Verification items for the finished model (mm, model axes). A direction names the side the tool comes from. Give positions to 0.01 mm unless a question says otherwise; leave off trailing zeros. Write each loop counter-clockwise with the first axis right and the second up, starting at its lowest first coordinate (ties: lowest second). Pieces come first, ordered by that corner, then holes. Notation, with made-up numbers: (17, 7.5) -> (36, 7.5) arc R18 cw to (36, 28.5) -> close; hole circle Ø8 at (0.5, 55.5). An arc over 180 degrees is marked (long way). Answer as CSV lines item,"result".
```python
from build123d import *

# Parameters (mm, degrees)
SKETCH1_R           = 2
BOSS_EXTRUDE1_DEPTH = 6


with BuildPart() as part:
    # Sketch1 → Boss-Extrude1 (new body)
    with BuildSketch(Plane(origin=(0, 0, 0), x_dir=(1, 0, 0), z_dir=(0, 1, 0))):
        Polygon((-45, 15), (-45, -10), (-50, -10), (-50, -15), (-45, -15), (-45, -20), (-50, -20), (-50, -30), (-45, -30), (-45, -35), (-50, -35), (-50, -40), (-45, -40), (45, -40), (50, -40), (50, -35), (45, -35), (45, -33), (45, -30), (50, -30), (50, -20), (45, -20), (45, -15), (50, -15), (50, -10), (45, -10), (45, 15), (19, 35), (-19, 35), align=None)
        with Locations(Location((15, 0, 0), (0, 0, 270))):
            Circle(SKETCH1_R, mode=Mode.SUBTRACT)
        with Locations(Location((-15, 0, 0), (0, 0, 270))):
            Circle(SKETCH1_R, mode=Mode.SUBTRACT)
        with Locations(Location((15, 27, 0), (0, 0, 270))):
            Circle(SKETCH1_R, mode=Mode.SUBTRACT)
        with Locations(Location((-15, 27, 0), (0, 0, 270))):
            Circle(SKETCH1_R, mode=Mode.SUBTRACT)
        with Locations(Location((0, 30, 0), (0, 0, 270))):
            Circle(SKETCH1_R, mode=Mode.SUBTRACT)
        with Locations(Location((-36, -12, 0), (0, 0, 270))):
            Circle(SKETCH1_R, mode=Mode.SUBTRACT)
        with Locations(Location((36, -12, 0), (0, 0, 270))):
            Circle(SKETCH1_R, mode=Mode.SUBTRACT)
        with BuildLine():
            Line((7, -30.5), (23, -30.5))
            ThreePointArc((23, -30.5), (25.5, -33), (23, -35.5))
            Line((23, -35.5), (7, -35.5))
            ThreePointArc((7, -35.5), (4.5, -33), (7, -30.5))
        make_face(mode=Mode.SUBTRACT)
    extrude(amount=BOSS_EXTRUDE1_DEPTH)


solid = part.part
```
1) Section check C-C (x = -15). Record the boundary of the cut face in (y, z).
Reported:
outline,"(0, -35) -> (6, -35) -> (6, -29) -> (0, -29) -> close; (0, -25) -> (6, -25) -> (6, -2) -> (0, -2) -> close; (0, 2) -> (6, 2) -> (6, 40) -> (0, 40) -> close"
2) Scan lines: line 1 along X through (y, z) = (3, 0); line 2 along Z through (x, y) = (-13.5, 5.2); line 3 along X through (y, z) = (2.75, 12). Record each from-to range of solid material in increasing order.
Reported:
line 1,"-45 to -17, -13 to 13, 17 to 45"
line 2,"-35 to -28.32, -25.68 to -1.32, 1.32 to 40"
line 3,"-50 to -38, -34 to 34, 38 to 50"
3) Section check D-D (z = 0). Record the boundary of the cut face in (x, y).
Reported:
outline,"(-45, 0) -> (-17, 0) -> (-17, 6) -> (-45, 6) -> close; (-13, 0) -> (13, 0) -> (13, 6) -> (-13, 6) -> close; (17, 0) -> (45, 0) -> (45, 6) -> (17, 6) -> close"
4) Tool access check on faces 1 (the flat face through (47, 3, 30)), 2 (the flat face through (48, 3, 10)), 3 (the flat face through (15, 3, 35.5)), 4 (the flat face through (-45, 3, 17)). Record the directions out of +Z, -Z, +X, -X, +Y, -Y that give a thin tool (end or side, any length) a straight path to the whole face; none if there is none.
Reported:
face 1,"+X, +Y, -Y"
face 2,"-Z, +X, +Y, -Y"
face 3,"+Y, -Y"
face 4,"-X, +Y, -Y"
5) Section check A-A (z = 33). Record the boundary of the cut face in (x, y).
Reported:
outline,"(-45, 0) -> (4.5, 0) -> (4.5, 6) -> (-45, 6) -> close; (25.5, 0) -> (45, 0) -> (45, 6) -> (25.5, 6) -> close"
6) Draft check along Z on faces 5 (the flat face through (-47, 3, 10)), 6 (the flat face through (-50, 3, 25)), 7 (the cylindrical face through (4.5, 3, 33.1)). Enter one of: +Z half, -Z half, draft (parallel to the pull), parting line (faces both ways), or undercut.
Reported:
face 5,"-Z half"
face 6,"draft"
face 7,"undercut"
7) Section check B-B (x = 15). Record the boundary of the cut face in (y, z), and give its area (3 significant figures).
Reported:
outline,"(0, -35) -> (6, -35) -> (6, -29) -> (0, -29) -> close; (0, -25) -> (6, -25) -> (6, -2) -> (0, -2) -> close; (0, 2) -> (6, 2) -> (6, 30.5) -> (0, 30.5) -> close; (0, 35.5) -> (6, 35.5) -> (6, 40) -> (0, 40) -> close"
area,"372 mm²"
8) Depth check by flat-ended pin: pin 1 (1.5 mm diameter, centred on y = 3, z = 18.5, fed in from -X); pin 2 (1.8 mm diameter, centred on y = 2.5, z = -5.5, fed in from +X); pin 3 (2.5 mm diameter, centred on x = 47, y = 3.5, fed in from -Z); pin 4 (2 mm diameter, centred on x = -18.5, z = 26.5, fed in from -Y). Enter the tip coordinate at first touch or a pass-through.
Reported:
pin 1,"x = -45"
pin 2,"x = 45"
pin 3,"z = 10"
pin 4,"y = 0"
